```python
from build123d import *

# Parameters (mm, degrees)
F1_DEPTH = 40
F2_SIZE  = 5
F3_R     = 5
F4_R     = 1.99999


# Not quite as in the source:
# - a fillet or chamfer is up to 0.001 mm smaller than in the source, because OpenCascade refuses the exact size


with BuildPart() as f1:
    # F0 (on Front) → F1 (new body)
    with BuildSketch(Plane.XZ):
        Polygon((-13, 36.2413817516), (-15, 36.2413817516), (-15, -28.7586182484), (0, -28.7586182484), (0, -18.7586182484), (-13, -18.7586182484), align=None)
        Polygon((0, 36.2413817516), (0, 56.2413817516), (-15, 56.2413817516), (-15, 36.2413817516), (-13, 36.2413817516), align=None)
    extrude(amount=F1_DEPTH)

    # F2
    f2_edges = [f1.edges().sort_by_distance(p)[0] for p in [
        (-13, -20, -18.758618),
        (-13, -20, 36.241382),
    ]]
    chamfer(f2_edges, length=F2_SIZE)

    # F3
    f3_edges = [f1.edges().sort_by_distance(p)[0] for p in [
        (-15, -20, 56.241382),
    ]]
    fillet(f3_edges, radius=F3_R)

    # F4 (radius 2 in the source; OpenCascade refuses exactly that, so slightly less here)
    f4_edges = [f1.edges().sort_by_distance(p)[0] for p in [
        (-15, 0, 11.241382),
        (-15, -20, 51.241382),
        (-15, -20, -28.758618),
        (-15, -40, 11.241382),
    ]]
    fillet(f4_edges, radius=F4_R)


solid = f1.part
```
Verification items for the finished model (mm, model axes). A direction names the side the tool comes from. Coordinates: 2 decimals unless noted, no trailing zeros. Write each loop counter-clockwise with the first axis right and the second up, starting at its lowest first coordinate (ties: lowest second). Pieces come first, ordered by that corner, then holes. Notation, with made-up numbers: M 60,-14.75 L 101,-14.75 A27 cw 101,8.25 Z; hole C 58,25 d2. An arc over 180 degrees is marked long. Answer as a JSON object with one key per item and string values. Group by question number.
(1) Cross-section at A-A, the plane x = -5.25. Record the cut outline in (y, z).
(2) Material ranges on line 1 (Z direction, x = -1, y = -5.5); line 2 (Z direction, x = -8.5, y = -20); line 3 (X direction, y = -30.5, z = 22.5), recorded low to high.
(3) Cross-section at B-B, the plane y = -4. Record the cut outline in (x, z).
(4) Cross-section at D-D, the plane z = -15.5. Record the cut outline in (x, y), and give its area (3 significant figures).
(5) Tool access check on faces 5 (the face through (-14.43, -20.28, -28.157)), 6 (the face through (-10.54, -19.72, -16.22)). Record the directions out of +Z, -Z, +X, -X, +Y, -Y that give a thin tool (end or side, any length) a straight path to the whole face; none if there is none.
(6) Gauge pin test, flat ends, axial feed: pin 1 (2 mm diameter, centred on x = -11.5, y = -35, fed in from +Z); pin 2 (6 mm diameter, centred on y = -22, z = -6.5, fed in from +X). Record the tip position at first contact, or that the pin passes through.
(7) Release check for a two-part mould opening along Z. For faces 1 (the face through (-4, -20, -18.759)), 2 (the face through (-14.4, -0.57, 10.68)), 3 (the face through (-5.07, -39.4, 55.67)), 4 (the face through (-10.46, -19.72, 33.78)) record: +Z half, -Z half, draft (parallel to the pull), parting line (faces both ways), or undercut.
Reply:
{
 "1": {"outline": "M -40,-28.76 L 0,-28.76 L 0,-18.76 L -40,-18.76 Z; M -40,36.24 L 0,36.24 L 0,54.24 A2 ccw -2,56.24 L -38,56.24 A2 ccw -40,54.24 Z"},
 "2": {"line 1": "-28.76 to -18.76, 36.24 to 56.24", "line 2": "-28.76 to -18.26, 35.74 to 56.24", "line 3": "-15 to -13"},
 "3": {"outline": "M -15,-26.76 A2 ccw -13,-28.76 L 0,-28.76 L 0,-18.76 L -8,-18.76 L -13,-13.76 L -13,31.24 L -8,36.24 L 0,36.24 L 0,56.24 L -10,56.24 A5 ccw -15,51.24 Z"},
 "4": {"outline": "M -15,-38 A2 ccw -13,-40 L -11.26,-40 L -11.26,0 L -13,0 A2 ccw -15,-2 Z", "area": "148 mm²"},
 "5": {"face 5": "-Z, -X, +Y, -Y", "face 6": "+X, +Y, -Y"},
 "6": {"pin 1": "z = 56.22", "pin 2": "x = -13"},
 "7": {"face 1": "undercut", "face 2": "draft", "face 3": "+Z half", "face 4": "undercut"}
}
